```python
from build123d import *

# Parameters (mm, degrees)
SZKIC3_R                   = 40
SZKIC3_W                   = 25
SZKIC3_H                   = 30
WYTNIJ_WYCI_GNI_CIE1_DEPTH = 30
ZAOKR_GLENIE1_R            = 10
SZYK_KO_OWY1_COUNT         = 4
ZAOKR_GLENIE2_R            = 5
SFAZOWANIE2_SIZE           = 5


with BuildPart() as part:
    # Szkic2 → Obrót1 (revolve)
    with BuildSketch(Plane.XY):
        Polygon((-293.485716032, 20), (46.514283968, 20), (46.514283968, 80), (-33.485716032, 80), (-33.485716032, 40), (-293.485716032, 40), align=None)
    revolve(axis=Axis((-88.99, 0, 0), (1, 0, 0)))

    # Szkic3 → Wytnij-wyciągnięcie1 (cut)
    with BuildSketch(Plane(origin=(46.514283968, 0, 0), x_dir=(0, 0, -1), z_dir=(1, 0, 0))):
        Circle(SZKIC3_R)
        with Locations((0, 75)):
            Rectangle(SZKIC3_W, SZKIC3_H)
    wytnij_wyci_gni_cie1 = extrude(amount=-WYTNIJ_WYCI_GNI_CIE1_DEPTH, mode=Mode.SUBTRACT)

    # Zaokrąglenie1
    zaokr_glenie1_edges = [part.edges().sort_by_distance(p)[0] for p in [
        (16.514283968, 60, 0),
    ]]
    fillet(zaokr_glenie1_edges, radius=ZAOKR_GLENIE1_R)

    # Szyk kołowy1: Wytnij-wyciągnięcie1 ×4 about axis
    szyk_ko_owy1_axis = Axis((0, 0, 0), (1, 0, 0))
    for i in range(1, SZYK_KO_OWY1_COUNT):
        add(wytnij_wyci_gni_cie1.rotate(szyk_ko_owy1_axis, i * 360 / SZYK_KO_OWY1_COUNT), mode=Mode.SUBTRACT)

    # Zaokrąglenie2
    zaokr_glenie2_edges = [part.edges().sort_by_distance(p)[0] for p in [
        (-33.485716032, -40, 0),
        (-33.485716032, -80, 0),
    ]]
    fillet(zaokr_glenie2_edges, radius=ZAOKR_GLENIE2_R)

    # Sfazowanie2
    sfazowanie2_edges = [part.edges().sort_by_distance(p)[0] for p in [
        (-293.485716032, -40, 0),
        (-293.485716032, -20, 0),
    ]]
    chamfer(sfazowanie2_edges, length=SFAZOWANIE2_SIZE)


solid = part.part
```
Here's how the part is built. I have some questions about the finished solid (model axes, mm). A direction names the side the tool comes from. Give positions to 0.01 mm unless a question says otherwise; leave off trailing zeros. Order: outer loops, then holes, each group sorted by start corner. A loop starts at its lowest first (then second) coordinate and runs counter-clockwise, first axis right, second up. Notation, with made-up numbers: M 72,28 L 127,28 A16 cw 127,50 Z; hole C 32.5,15.25 d10. An arc over 180 degrees is marked long. Use a Markdown table: item, result. Add a question column.
1. Suppose I cut it at A-A (y = 0). List the corners of the cut face in (x, z) for me.
2. Suppose I cut it at C-C (x = -199). List the corners of the cut face in (y, z) for me.
3. For pin 1 Ø3 at (y, z) = (60, 48) entering from -X; pin 2 Ø6 at (y, z) = (-3.5, 71.5) entering from +X; pin 3 Ø21 at (x, z) = (26, -74) entering from +Y, each with a flat end and sliding along its axis, tell me the tip position at first contact or that it passes through.
4. Suppose I cut it at D-D (x = -11.5). List the corners of the cut face in (y, z) for me, and give its area (3 significant figures).
5. I need wall thicknesses on probe 1 along Y at (x, z) = (29.5, 0); probe 2 along Z at (x, y) = (-226.5, 0). Which ranges of each line are inside material? Lowest first, please. Write a range as from..to.
6. On a 3-axis mill with a long thin cutter (end or side, diameter ignored), from which of +Z, -Z, +X, -X, +Y, -Y can I reach the whole of each face in a straight line? I mean faces 1 (the flat face through (32, 0, 60)), 2 (the flat face through (32, 69, -12.5)), 3 (the flat face through (32, -60, 0)), 4 (the flat face through (16.514, 18.3, 9.4)), 5 (the cylindrical face through (-165.24, -8.67, -39.05)). Say none if no direction works.
Results list:
| question | item | result |
|---|---|---|
| 1 | outline | M -293.49,-35 L -288.49,-40 L -38.49,-40 A5 cw -33.49,-45 L -33.49,-75 A5 ccw -28.49,-80 L 16.51,-80 L 16.51,-60 L 46.51,-60 L 46.51,-40 L 16.51,-40 L 16.51,-20 L -288.49,-20 L -293.49,-25 Z; M -293.49,25 L -288.49,20 L 16.51,20 L 16.51,40 L 46.51,40 L 46.51,60 L 16.51,60 L 16.51,80 L -28.49,80 A5 ccw -33.49,75 L -33.49,45 A5 cw -38.49,40 L -288.49,40 L -293.49,35 Z |
| 2 | outline | C 0,0 d80; hole C 0,0 d40 |
| 3 | pin 1 | stops at x = -33.47 |
| 3 | pin 2 | stops at x = 16.51 |
| 3 | pin 3 | stops at y = 48.66 |
| 4 | outline | C 0,0 d160; hole C 0,0 d40 |
| 4 | area | 18,800 mm² |
| 5 | probe 1 | y = -60..-40, 40..60 |
| 5 | probe 2 | z = -40..-20, 20..40 |
| 6 | face 1 | +Z, +X |
| 6 | face 2 | +X, +Y |
| 6 | face 3 | +X, -Y |
| 6 | face 4 | +X |
| 6 | face 5 | -X |
